Can you work these out from the model? Positions are in its coordinate system, mm. Face numbers are marked on the shaded views. Coordinates: 2 decimals unless noted, no trailing zeros. Order: outer loops, then holes, each group sorted by start corner. A loop starts at its lowest first (then second) coordinate and runs counter-clockwise, first axis right, second up. Notation, with made-up numbers: (-35.75, 64.5) - (-2.75, 64.5) arc R21 ccw to (-2.75, 99.5) - close; hole circle Ø1 at (-0.5, 36). An arc over 180 degrees is marked (long way). Return JSON: item names as keys, results as strings. Group by question number.
1) For pin 1 Ø2 at (y, z) = (9.5, 0) entering from +X; pin 2 Ø1.2 at (y, z) = (4, -2.5) entering from +X; pin 3 Ø3 at (y, z) = (2, 23.5) entering from -X, each with a flat end and sliding along its axis, tell me the tip position at first contact or that it passes through.
2) If we mould it in two halves opening along Z, with no side actions, what happens to the marked faces 1, 2 and 3? For each: pulls with the +Z half, pulls with the -Z half, needs draft (parallel to the pull), parting line crosses it, or undercut.
3) Imagine slicing it at C-C (z = -13). Give the number of separate pieces and of enclosed holes in the cut face, and give its area (3 significant figures).
4) Imagine slicing it at B-B (x = 6). Write out the boundary of the cut face in (y, z), and give its area (3 significant figures).
5) If I drill on line 1 along Z through (x, y) = (0, 0.5); line 2 along X through (y, z) = (0.85, 23); line 3 along Z through (x, y) = (0, 7.75), over which ranges is the centre line in solid material (lowest first)?
6) Imagine slicing it at A-A (z = 23). Write out the boundary of the cut face in (x, y), and give its area (3 significant figures).
7) Imagine slicing it at D-D (y = 13). Write out the boundary of the cut face in (x, z).
Autodesk Inventor part; units mm, degrees
ref_plane "YZ Plane" through (0, 0, 0) normal (1, 0, 0) x (0, 1, 0)
ref_plane "XZ Plane" through (0, 0, 0) normal (0, 1, 0) x (-1, 0, 0)
ref_plane "XY Plane" through (0, 0, 0) normal (0, 0, 1) x (1, 0, 0)
sketch "Sketch1" plane through (0, 0, 0) normal (0, 1, 0) x (-1, 0, 0)
  line L0 (12.25, -7.0725) -> (0, -14.1451)
  line L1 (0, -14.1451) -> (-12.25, -7.0725)
  line L2 (-12.25, -7.0725) -> (-12.25, 7.0725)
  line L3 (-12.25, 7.0725) -> (0, 14.1451)
  line L4 (0, 14.1451) -> (12.25, 7.0725)
  line L5 (12.25, 7.0725) -> (12.25, -7.0725)
  circle A0 centre (0, 0) radius 16.5
  dimension "d0" = 12.25
  dimension "d1" = 33
extrude "Extrusion1" add sketch "Sketch1" along normal blind 5
sketch "Sketch2" plane through (0, 0, 0) normal (0, -1, 0) x (1, 0, 0)
  line L0 (0, 14.1451) -> (-12.25, 7.0725)
  line L1 (-12.25, 7.0725) -> (-12.25, -7.0725)
  line L2 (-12.25, -7.0725) -> (0, -14.1451)
  line L3 (0, -14.1451) -> (12.25, -7.0725)
  line L4 (12.25, -7.0725) -> (12.25, 7.0725)
  line L5 (12.25, 7.0725) -> (0, 14.1451)
  point P0 (0, 0)
extrude "Extrusion2" add sketch "Sketch2" against normal blind 2.5
sketch "Sketch3" plane through (0, 0, 0) normal (0, -1, 0) x (1, 0, 0)
  circle A0 centre (0, 0) radius 10
  dimension "d6" = 20
extrude "Extrusion3" cut sketch "Sketch3" against normal blind 2.5
sketch "Sketch4" plane through (0, 5, 0) normal (0, 1, 0) x (1, 0, 0)
  circle A0 centre (0, 0) radius 14.5
  circle A1 centre (0, 0) radius 16.5
  dimension "d9" = 29
extrude "Extrusion4" add sketch "Sketch4" along normal blind 10
sketch "Sketch5" plane through (0, 0, 0) normal (0, -1, 0) x (1, 0, 0)
  circle A0 centre (0, 0) radius 16.5
  arc A1 (14.2894, -8.25) -> (0, 16.5) centre (0, 0) ccw
  line L0 (0, 0) -> (14.2894, -8.25) construction
  line L1 (0, 0) -> (0, 16.5) construction
  arc A2 (0, 16.5) -> (-14.2894, -8.25) centre (0, 0) ccw
  line L2 (0, 0) -> (-14.2894, -8.25) construction
  line L3 (0, 0) -> (0, 16.5) construction
  circle A3 centre (0, 0) radius 14.5
  line L4 (0, 14.5) -> (4, 14.5)
  line L5 (4, 14.5) -> (4, 26.5)
  line L6 (4, 26.5) -> (-4, 26.5)
  line L7 (0, 14.5) -> (-4, 14.5)
  line L8 (-4, 14.5) -> (-4, 26.5)
  line L9 (0, 16.5) -> (0, 23)
  circle A4 centre (0, 23) radius 2.5
  line L10 (-12.5574, -7.25) -> (-10.5574, -10.7141)
  line L11 (-12.5574, -7.25) -> (-14.5574, -3.7859)
  line L12 (-14.2894, -8.25) -> (-19.9186, -11.5)
  line L13 (-10.5574, -10.7141) -> (-20.9497, -16.7141)
  circle A5 centre (-19.9186, -11.5) radius 2.5
  line L14 (-24.9497, -9.7859) -> (-20.9497, -16.7141)
  line L15 (-14.5574, -3.7859) -> (-24.9497, -9.7859)
  line L16 (12.5574, -7.25) -> (14.5574, -3.7859)
  line L17 (12.5574, -7.25) -> (10.5574, -10.7141)
  line L18 (14.2894, -8.25) -> (19.9186, -11.5)
  line L19 (14.5574, -3.7859) -> (24.9497, -9.7859)
  circle A6 centre (19.9186, -11.5) radius 2.5
  line L20 (20.9497, -16.7141) -> (24.9497, -9.7859)
  line L21 (10.5574, -10.7141) -> (20.9497, -16.7141)
  point P0 (11.8632, -11.468)
  point P1 (15.8632, -4.5398)
  point P2 (-15.8632, -4.5398)
  point P3 (-11.8632, -11.468)
  point P4 (4, 16.0078)
  point P5 (-4, 16.0078)
  dimension "d12" = 120
  dimension "d13" = 120
  dimension "d14" = 4
  dimension "d15" = 12
  dimension "d16" = 8
  dimension "d17" = 4
  dimension "d18" = 6.5
  dimension "d19" = 5
  dimension "d22" = 360
extrude "Extrusion5" add sketch "Sketch5" against normal blind 2.5 contours A0 L8 L6 L5 | L19 L20 L21 A0 | A0 L13 L14 L15
sketch "Sketch6" plane through (0, 15, 0) normal (0, 1, 0) x (1, 0, 0)
  circle A0 centre (0, 0) radius 16
  circle A1 centre (0, 0) radius 17.8656
  dimension "d31" = 32
extrude "Extrusion6" cut sketch "Sketch6" against normal up to surface (12.5 mm away)
properties part number "receptor_manguera"
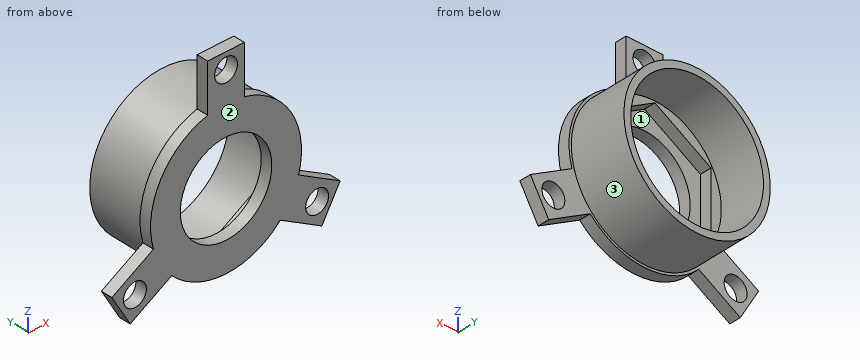
Calculated:
{
 "1": {"pin 1": "x = 16", "pin 2": "x = 15.89", "pin 3": "x = -4"},
 "2": {"face 1": "undercut", "face 2": "needs draft", "face 3": "parting line crosses it"},
 "3": {"separate pieces": "5", "enclosed holes": "0", "area": "169 mm2"},
 "4": {"outline": "(0, -15.37) - (2.5, -15.37) - (2.5, -14.83) - (15, -14.83) - (15, -13.2) - (5, -13.2) - (5, -10.68) - (2.5, -10.68) - (2.5, -8) - (0, -8) - close; (0, 8) - (2.5, 8) - (2.5, 10.68) - (5, 10.68) - (5, 13.2) - (15, 13.2) - (15, 14.83) - (2.5, 14.83) - (2.5, 15.37) - (0, 15.37) - close", "area": "90.2 mm2"},
 "5": {"line 1": "-16.5 to -10, 10 to 20.5, 25.5 to 26.5", "line 2": "-4 to -2.5, 2.5 to 4", "line 3": "-16 to -14.5, 14.5 to 16"},
 "6": {"outline": "(-4, 0) - (-2.5, 0) - (-2.5, 2.5) - (-4, 2.5) - close; (2.5, 0) - (4, 0) - (4, 2.5) - (2.5, 2.5) - close", "area": "7.50 mm2"},
 "7": {"outline": "circle Ø32 at (0, 0); hole circle Ø29 at (0, 0)"}
}
